Check sheet for the modelled part. Datum: model origin and axes. Units: mm. A direction names the side the tool comes from. Round coordinates to 2 decimals unless told otherwise and drop trailing zeros. Order: outer loops, then holes, each group sorted by start corner. A loop starts at its lowest first (then second) coordinate and runs counter-clockwise, first axis right, second up. Notation, with made-up numbers: (14, -22) -> (70, -22) arc R17 cw to (70, 11) -> close; hole circle Ø6 at (3.5, 54). An arc over 180 degrees is marked (long way). Answer in a Markdown table with one row per item.
from build123d import *

# Parameters (mm, degrees)
F1_W     = 80
F1_H     = 55
F2_DEPTH = 3.175
F3_W     = 3.175
F3_H     = 15
F3_W_2   = 15
F3_H_2   = 3.175
F3_W_3   = 3.75
F3_H_3   = 3.1
F3_W_4   = 2.5
F3_H_4   = 1.1
F3_W_5   = 2.75
F4_DEPTH = 3.176


with BuildPart() as f2:
    # F1 (on Right) → F2 (new body)
    with BuildSketch(Plane.YZ):
        Rectangle(F1_W, F1_H)
    extrude(amount=F2_DEPTH)

    # F3 (on face) → F4 (cut, through all)
    with BuildSketch(Plane.YZ.offset(3.175)):
        with Locations((38.4125, 0)):
            Rectangle(F3_W, F3_H)
        with Locations((-17.5, -25.9125)):
            Rectangle(F3_W_2, F3_H_2)
        with Locations((17.5, -25.9125)):
            Rectangle(F3_W_2, F3_H_2)
        with Locations((-17.5, 25.9125)):
            Rectangle(F3_W_2, F3_H_2)
        with Locations((17.5, 25.9125)):
            Rectangle(F3_W_2, F3_H_2)
        with Locations((-34.95, 0)):
            Rectangle(F3_W_3, F3_H_3)
        Polygon((-36.825, -7.5), (-36.825, -1.55), (-36.825, 1.55), (-36.825, 7.5), (-40, 7.5), (-40, -7.5), align=None)
        with Locations((-31.825, 0)):
            Rectangle(F3_W_4, F3_H_3)
        with Locations((-31.825, -2.1)):
            Rectangle(F3_W_4, F3_H_4)
        with Locations((-29.2, 0)):
            Rectangle(F3_W_5, F3_H_3)
        with Locations((-31.825, 2.1)):
            Rectangle(F3_W_4, F3_H_4)
    extrude(amount=-F4_DEPTH, mode=Mode.SUBTRACT)


solid = f2.part
Item 1: Scan lines: line 1 (Y direction, x = 2.8, z = -25); line 2 (Z direction, x = 1.8, y = -29.5); line 3 (Y direction, x = 3.05, z = 3) (3 decimals). Record each from-to range of solid material in increasing order. Write a range as [from, to].
Result sheet:
| item | result |
|---|---|
| line 1 | y = [-40, -25], [-10, 10], [25, 40] |
| line 2 | z = [-27.5, -1.55], [1.55, 27.5] |
| line 3 | y = [-36.825, 36.825] |
Item 2: Depth check by flat-ended pin: P1, Ø1, axis at x = 2, z = 3.5, coming from the +Y side (3 decimals); P2, Ø1, axis at x = 2, z = 4, coming from the -Y side (3 decimals). Enter the tip coordinate at first touch or a pass-through.
Result sheet:
| item | result |
|---|---|
| P1 | stops at y = 36.825 |
| P2 | stops at y = -36.825 |
Item 3: Cross-section at A-A (y = 22.5). Record the boundary of the cut face in (x, z) (3 decimals).
Result sheet:
| item | result |
|---|---|
| outline | (0, -24.325) -> (3.175, -24.325) -> (3.175, 24.325) -> (0, 24.325) -> close |
Item 4: Set-up check for faces 1 (the flat face through (2, 40, 17)), 2 (the flat face through (2, -33, 27.5)), 3 (the flat face through (2, 17, 24.325)), 4 (the flat face through (2, 25, -26)), 5 (the flat face through (2, -38, 7.5)): record each of +Z, -Z, +X, -X, +Y, -Y from which the full face is reachable in a straight line by a thin tool's end or side.
Result sheet:
| item | result |
|---|---|
| face 1 | +Z, -Z, +X, -X, +Y |
| face 2 | +Z, +X, -X, +Y, -Y |
| face 3 | +Z, +X, -X |
| face 4 | -Z, +X, -X |
| face 5 | +X, -X, -Y |
Item 5: Cross-section at B-B (z = -4.5). Record the boundary of the cut face in (x, y) (3 decimals), and give its area (3 significant figures).
Result sheet:
| item | result |
|---|---|
| outline | (0, -36.825) -> (3.175, -36.825) -> (3.175, 36.825) -> (0, 36.825) -> close |
| area | 234 mm^2 |
Item 6: Mould release check, pull along Y, two halves, no side actions. Record for faces 6 (the flat face through (2, -36.825, 4)), 7 (the flat face through (2, -25, 26)), 8 (the flat face through (2, 0, -27.5)): pulls with the +Y half, pulls with the -Y half, needs draft (parallel to the pull), parting line crosses it, or undercut.
Result sheet:
| item | result |
|---|---|
| face 6 | pulls with the -Y half |
| face 7 | undercut |
| face 8 | needs draft |
